Here's how the part is built. I have some questions about the finished solid (model axes, mm). A direction names the side the tool comes from. Round coordinates to 2 decimals unless told otherwise and drop trailing zeros. Order: outer loops, then holes, each group sorted by start corner. A loop starts at its lowest first (then second) coordinate and runs counter-clockwise, first axis right, second up.
Autodesk Inventor part; units mm, degrees
ref_plane "YZ Plane" through (0, 0, 0) normal (1, 0, 0) x (0, 1, 0)
ref_plane "XZ Plane" through (0, 0, 0) normal (0, 1, 0) x (-1, 0, 0)
ref_plane "XY Plane" through (0, 0, 0) normal (0, 0, 1) x (1, 0, 0)
sketch "Sketch1" plane through (0, 0, 0) normal (0, 0, 1) x (1, 0, 0)
  circle A0 centre (0, 0) radius 3.5
  line L0 (77.9423, 0) -> (38.9711, -67.5)
  line L1 (38.9711, -67.5) -> (-38.9711, -67.5)
  line L2 (-38.9711, -67.5) -> (-77.9423, 0)
  line L3 (-77.9423, 0) -> (-38.9711, 67.5)
  line L4 (-38.9711, 67.5) -> (38.9711, 67.5)
  line L5 (38.9711, 67.5) -> (77.9423, 0)
  circle A1 centre (22.5, 0) radius 2.25
  circle A2 centre (54, 0) radius 2
  circle A3 centre (15.9099, 15.9099) radius 2.25
  circle A4 centre (0, 22.5) radius 2.25
  circle A5 centre (-15.9099, 15.9099) radius 2.25
  circle A6 centre (-22.5, 0) radius 2.25
  circle A7 centre (-15.9099, -15.9099) radius 2.25
  circle A8 centre (0, -22.5) radius 2.25
  circle A9 centre (15.9099, -15.9099) radius 2.25
  circle A10 centre (46.7654, 27) radius 2
  circle A11 centre (27, 46.7654) radius 2
  circle A12 centre (0, 54) radius 2
  circle A13 centre (-27, 46.7654) radius 2
  circle A14 centre (-46.7654, 27) radius 2
  circle A15 centre (-54, 0) radius 2
  circle A16 centre (-46.7654, -27) radius 2
  circle A17 centre (-27, -46.7654) radius 2
  circle A18 centre (0, -54) radius 2
  circle A19 centre (27, -46.7654) radius 2
  circle A20 centre (46.7654, -27) radius 2
  dimension "d0" = 7
  dimension "d1" = 135
  dimension "d2" = 22.5
  dimension "d3" = 4.5
  dimension "d4" = 4
  dimension "d5" = 54
  dimension "d8" = 360
  dimension "d12" = 360
extrude "Extrusion1" add sketch "Sketch1" along normal blind 30
sketch "Sketch2" plane through (0, 0, 30) normal (0, 0, 1) x (1, 0, 0)
  circle A0 centre (0, 0) radius 3.5
  circle A1 centre (0, 0) radius 49
  dimension "d16" = 98
extrude "Extrusion2" cut sketch "Sketch2" against normal blind 15
sketch "Sketch3" plane through (0, 0, 15) normal (0, 0, 1) x (1, 0, 0)
  circle A0 centre (0, 0) radius 33
  dimension "d19" = 66
extrude "Extrusion3" cut sketch "Sketch3" against normal blind 3
sketch "Sketch4" plane through (0, 0, 12) normal (0, 0, 1) x (1, 0, 0)
  circle A0 centre (0, 0) radius 16.5
  circle A1 centre (0, 0) radius 3.5
  dimension "d22" = 33
extrude "Extrusion4" add sketch "Sketch4" along normal blind 33
sketch "Sketch5" plane through (0, 0, 45) normal (0, 0, 1) x (1, 0, 0)
  circle A0 centre (8, 0) radius 2.5
  circle A1 centre (2.4721, 7.6085) radius 2.5
  circle A2 centre (-6.4721, 4.7023) radius 2.5
  circle A3 centre (-6.4721, -4.7023) radius 2.5
  circle A4 centre (2.4721, -7.6085) radius 2.5
  point P0 (0, 0)
  dimension "d25" = 5
  dimension "d26" = 8
  dimension "d29" = 360
extrude "Extrusion5" cut sketch "Sketch5" against normal through all
sketch "Sketch6" plane through (0, 0, 0) normal (0, 0, -1) x (-1, 0, 0)
  circle A0 centre (0, 0) radius 17.5
  dimension "d33" = 35
extrude "Extrusion6" cut sketch "Sketch6" against normal blind 5
sketch "Sketch10" plane through (0, 0, 0) normal (0, 0, -1) x (-1, 0, 0)
  circle A0 centre (22.5, 0) radius 2.25
  circle A1 centre (0, 0) radius 3.5
  circle A2 centre (0, 0) radius 20.25
  circle A3 centre (0, 0) radius 24.75
  circle A4 centre (0, 0) radius 16
  circle A5 centre (0, 0) radius 29
  line L0 (29, 0) -> (16, 0)
  dimension "d38" = 13
extrude "Extrusion7" cut sketch "Sketch10" against normal blind 5 contours L0 A0 | A2 | A3 | A5 | A0 L0
sketch "Sketch11" plane through (0, 0, 12) normal (0, 0, 1) x (1, 0, 0)
  circle A0 centre (0, 0) radius 16.5
  circle A1 centre (15.9099, -15.9099) radius 2.25
  circle A2 centre (0, -22.5) radius 2.25
  circle A3 centre (-15.9099, -15.9099) radius 2.25
  circle A4 centre (-22.5, 0) radius 2.25
  circle A5 centre (-15.9099, 15.9099) radius 2.25
  circle A6 centre (0, 22.5) radius 2.25
  circle A7 centre (15.9099, 15.9099) radius 2.25
  circle A8 centre (22.5, 0) radius 2.25
  circle A9 centre (0, 0) radius 33
extrude "Extrusion8" add sketch "Sketch11" along normal up to surface (3 mm away) from surface at 0
sketch "Sketch12" plane through (0, 0, 30) normal (0, 0, 1) x (1, 0, 0)
  circle A0 centre (0, 0) radius 49
  circle A1 centre (46.7654, -27) radius 2
  circle A2 centre (27, -46.7654) radius 2
  circle A3 centre (0, -54) radius 2
  circle A4 centre (-27, -46.7654) radius 2
  circle A5 centre (-46.7654, -27) radius 2
  circle A6 centre (-54, 0) radius 2
  circle A7 centre (-46.7654, 27) radius 2
  circle A8 centre (-27, 46.7654) radius 2
  circle A9 centre (0, 54) radius 2
  circle A10 centre (27, 46.7654) radius 2
  circle A11 centre (46.7654, 27) radius 2
  circle A12 centre (54, 0) radius 2
  line L0 (38.9711, -67.5) -> (77.9423, 0)
  line L1 (77.9423, 0) -> (38.9711, 67.5)
  line L2 (38.9711, 67.5) -> (-38.9711, 67.5)
  line L3 (-38.9711, 67.5) -> (-77.9423, 0)
  line L4 (-77.9423, 0) -> (-38.9711, -67.5)
  line L5 (-38.9711, -67.5) -> (38.9711, -67.5)
extrude "Extrusion9" cut sketch "Sketch12" against normal blind 1
sketch "Sketch14" plane through (0, 0, 15) normal (0, 0, 1) x (1, 0, 0)
  circle A0 centre (0, 0) radius 3.5
  circle A1 centre (0, 0) radius 33
  circle A2 centre (15.9099, -15.9099) radius 2.25
  circle A3 centre (0, -22.5) radius 2.25
  circle A4 centre (-15.9099, -15.9099) radius 2.25
  circle A5 centre (-22.5, 0) radius 2.25
  circle A6 centre (-15.9099, 15.9099) radius 2.25
  circle A7 centre (0, 22.5) radius 2.25
  circle A8 centre (15.9099, 15.9099) radius 2.25
  circle A9 centre (22.5, 0) radius 2.25
  circle A10 centre (0, 0) radius 16.5
  circle A11 centre (0, 0) radius 49
  dimension "d45" = 66
extrude "Extrusion10" cut sketch "Sketch14" against normal blind 4 contours A11
sketch "Sketch15" plane through (0, 0, 29) normal (0, 0, 1) x (1, 0, 0)
  circle A0 centre (0, 0) radius 49 construction
  circle A1 centre (54, 0) radius 2 construction
  circle A2 centre (46.7654, 27) radius 2 construction
  circle A3 centre (27, 46.7654) radius 2 construction
  circle A4 centre (0, 54) radius 2 construction
  circle A5 centre (-27, 46.7654) radius 2 construction
  circle A6 centre (-46.7654, 27) radius 2 construction
  circle A7 centre (-54, 0) radius 2 construction
  circle A8 centre (-46.7654, -27) radius 2 construction
  circle A9 centre (-27, -46.7654) radius 2 construction
  circle A10 centre (0, -54) radius 2 construction
  circle A11 centre (27, -46.7654) radius 2 construction
  circle A12 centre (46.7654, -27) radius 2 construction
  line L0 (77.9423, 0) -> (38.9711, -67.5)
  line L1 (38.9711, 67.5) -> (77.9423, 0)
  line L2 (-38.9711, 67.5) -> (38.9711, 67.5)
  line L3 (-77.9423, 0) -> (-38.9711, 67.5)
  line L4 (-38.9711, -67.5) -> (-77.9423, 0)
  line L5 (38.9711, -67.5) -> (-38.9711, -67.5)
  line L6 (36.0844, 62.5) -> (72.1688, 0)
  line L7 (72.1688, 0) -> (36.0844, -62.5)
  line L8 (36.0844, -62.5) -> (-36.0844, -62.5)
  line L9 (-36.0844, -62.5) -> (-72.1688, 0)
  line L10 (-72.1688, 0) -> (-36.0844, 62.5)
  line L11 (-36.0844, 62.5) -> (36.0844, 62.5)
  dimension "d48" = 5
extrude "Extrusion11" add sketch "Sketch15" along normal blind 0.8
sketch "Sketch16" plane through (0, 0, 0) normal (0, 0, -1) x (-1, 0, 0)
  circle A0 centre (0, 0) radius 29
  circle A1 centre (-46.7654, -27) radius 2
  circle A2 centre (-27, -46.7654) radius 2
  circle A3 centre (0, -54) radius 2
  circle A4 centre (27, -46.7654) radius 2
  circle A5 centre (46.7654, -27) radius 2
  circle A6 centre (54, 0) radius 2
  circle A7 centre (46.7654, 27) radius 2
  circle A8 centre (27, 46.7654) radius 2
  circle A9 centre (0, 54) radius 2
  circle A10 centre (-27, 46.7654) radius 2
  circle A11 centre (-46.7654, 27) radius 2
  circle A12 centre (-54, 0) radius 2
  line L0 (-77.9423, 0) -> (-38.9711, -67.5)
  line L1 (-38.9711, -67.5) -> (38.9711, -67.5)
  line L2 (38.9711, -67.5) -> (77.9423, 0)
  line L3 (77.9423, 0) -> (38.9711, 67.5)
  line L4 (38.9711, 67.5) -> (-38.9711, 67.5)
  line L5 (-38.9711, 67.5) -> (-77.9423, 0)
  line L6 (68.1273, 0) -> (34.0637, -59)
  line L7 (34.0637, -59) -> (-34.0637, -59)
  line L8 (-34.0637, -59) -> (-68.1273, 0)
  line L9 (-68.1273, 0) -> (-34.0637, 59)
  line L10 (-34.0637, 59) -> (34.0637, 59)
  line L11 (34.0637, 59) -> (68.1273, 0)
  dimension "d51" = 118
extrude "Extrusion12" cut sketch "Sketch16" along normal through all both and the other way through all contours L5 L4 L3 L2 L1 L0
sketch "Sketch17" plane through (0, 0, 0) normal (0, 0, -1) x (-1, 0, 0)
  circle A0 centre (0, -54) radius 2
  circle A1 centre (0, -54) radius 2
  circle A2 centre (27, -46.7654) radius 2
  circle A3 centre (46.7654, -27) radius 2
  circle A4 centre (54, 0) radius 2
  circle A5 centre (46.7654, 27) radius 2
  circle A6 centre (27, 46.7654) radius 2
  circle A7 centre (0, 54) radius 2
  circle A8 centre (-27, 46.7654) radius 2
  circle A9 centre (-46.7654, 27) radius 2
  circle A10 centre (-54, 0) radius 2
  circle A11 centre (-46.7654, -27) radius 2
  circle A12 centre (-27, -46.7654) radius 2
  point P0 (0, 0)
  dimension "d56" = 360
extrude "Extrusion13" add sketch "Sketch17" along normal up to surface (29 mm away) from surface at -29
sketch "Sketch18" plane through (0, 0, 0) normal (0, 0, -1) x (-1, 0, 0)
  line L0 (-46.188, 0) -> (-23.094, 40)
  line L1 (-23.094, 40) -> (23.094, 40)
  line L2 (23.094, 40) -> (46.188, 0)
  line L3 (46.188, 0) -> (23.094, -40)
  line L4 (23.094, -40) -> (-23.094, -40)
  line L5 (-23.094, -40) -> (-46.188, 0)
  line L6 (-19.0526, -33) -> (19.0526, -33)
  line L7 (19.0526, -33) -> (38.1051, 0)
  line L8 (38.1051, 0) -> (19.0526, 33)
  line L9 (19.0526, 33) -> (-19.0526, 33)
  line L10 (-19.0526, 33) -> (-38.1051, 0)
  line L11 (-38.1051, 0) -> (-19.0526, -33)
  line L12 (-34.0637, -59) -> (34.0637, -59)
  line L13 (34.0637, -59) -> (68.1273, 0)
  line L14 (68.1273, 0) -> (34.0637, 59)
  line L15 (34.0637, 59) -> (-34.0637, 59)
  line L16 (-34.0637, 59) -> (-68.1273, 0)
  line L17 (-68.1273, 0) -> (-34.0637, -59)
  circle A0 centre (0, 0) radius 29
  dimension "d60" = 80
  dimension "d61" = 7
extrude "Extrusion14" add sketch "Sketch18" along normal blind 13 contours L0 L1 L2 L3 L4 L5 | L17 L16 L15 L14 L13 L12
sketch "Sketch19" plane through (68.1273, 0, 29) normal (0.866, 0.5, 0) x (0, 0, -1)
  line L0 (29, 15.0111) -> (29, 53.1162)
  line L1 (29, 15.0111) -> (42, 15.0111)
  line L2 (42, 53.1162) -> (42, 15.0111)
  line L3 (29, 53.1162) -> (42, 53.1162)
  line L4 (38, 26.9926) -> (33, 41.1347) construction
  circle A0 centre (38, 26.9926) radius 2.5
  circle A1 centre (33, 41.1347) radius 2.5
  point P0 (29, 34.0637)
  point P1 (35.5, 15.0111)
  point P2 (35.5, 34.0637)
  point P3 (29, 34.0637)
  dimension "d64" = 15
  dimension "d65" = 5
  dimension "d66" = 5
  dimension "d72" = 5
extrude "Extrusion15" cut sketch "Sketch19" against normal blind 30 contours A0 | A1
pattern_circular "Circular Pattern1" count 6 over 360 about axis through (0, 0, 0) along (0, 0, 1) of "Extrusion15"
sketch "Sketch21" plane through (0, 0, 5) normal (0, 0, -1) x (-1, 0, 0)
  circle A0 centre (0, 17.5) radius 2
  circle A1 centre (-15.1554, -8.75) radius 2
  circle A2 centre (15.1554, -8.75) radius 2
  point P0 (0, 0)
  dimension "d74" = 4
  dimension "d75" = 17.5
  dimension "d78" = 360
extrude "Extrusion16" cut sketch "Sketch21" against normal through all
sketch "Sketch22" plane through (0, 0, 5) normal (0, 0, -1) x (-1, 0, 0)
  circle A0 centre (-15.1554, -8.75) radius 2
  circle A1 centre (0, 17.5) radius 2
  circle A2 centre (15.1554, -8.75) radius 2
  circle A3 centre (0, 0) radius 29
  circle A4 centre (-22.5, 0) radius 2.25
  circle A5 centre (-15.9099, 15.9099) radius 2.25
  circle A6 centre (0, 22.5) radius 2.25
  circle A7 centre (15.9099, 15.9099) radius 2.25
  circle A8 centre (22.5, 0) radius 2.25
  circle A9 centre (15.9099, -15.9099) radius 2.25
  circle A10 centre (0, -22.5) radius 2.25
  circle A11 centre (-15.9099, -15.9099) radius 2.25
  circle A12 centre (0, 0) radius 3.5
extrude "Extrusion17" cut sketch "Sketch22" against normal blind 5
sketch "Sketch23" plane through (0, 0, 10) normal (0, 0, -1) x (-1, 0, 0)
  circle A0 centre (0, 0) radius 3.5
  circle A1 centre (0, 0) radius 14.5
  dimension "d84" = 29
extrude "Extrusion18" [suppressed]
sketch "Sketch24" plane through (0, 0, 29) normal (0, 0, 1) x (1, 0, 0)
  line L0 (-34.0637, -59) -> (34.0637, -59)
  line L1 (34.0637, -59) -> (68.1273, 0)
  line L2 (68.1273, 0) -> (34.0637, 59)
  line L3 (34.0637, 59) -> (-34.0637, 59)
  line L4 (-34.0637, 59) -> (-68.1273, 0)
  line L5 (-68.1273, 0) -> (-34.0637, -59)
  circle A0 centre (0, 0) radius 49
extrude "Extrusion19" add sketch "Sketch24" along normal blind 1
sketch "Sketch25" plane through (0, 0, 10) normal (0, 0, -1) x (-1, 0, 0)
  circle A0 centre (-15.1554, -8.75) radius 2
  circle A1 centre (0, 17.5) radius 2
  circle A2 centre (15.1554, -8.75) radius 2
  point P0 (0, 0)
extrude "Extrusion20" add sketch "Sketch25" against normal up to surface (5 mm away) from surface at 0
sketch "Sketch26" plane through (0, 0, -13) normal (0, 0, -1) x (-1, 0, 0)
  circle A0 centre (-62, 0) radius 2.25
  circle A1 centre (-31, -53.6936) radius 2.25
  circle A2 centre (31, -53.6936) radius 2.25
  circle A3 centre (62, 0) radius 2.25
  circle A4 centre (31, 53.6936) radius 2.25
  circle A5 centre (-31, 53.6936) radius 2.25
  point P0 (0, 0)
  dimension "d91" = 4.5
  dimension "d92" = 62
  dimension "d95" = 360
extrude "Extrusion21" cut sketch "Sketch26" against normal through all
properties part number "AC05" material "ABS Plastic"
1. If we section it at D-D, the plane z = 33.5: Write out the boundary of the cut face in (x, y).
Evaluation:
outline: (-15.06, -6.75) arc R2 cw to (-13.38, -9.66) arc R16.5 ccw to (13.38, -9.66) arc R2 cw to (15.06, -6.75) arc R16.5 ccw to (1.68, 16.41) arc R2 cw to (-1.68, 16.41) arc R16.5 ccw to start; hole circle Ø5 at (-6.47, -4.7); hole circle Ø5 at (-6.47, 4.7); hole circle Ø7 at (0, 0); hole circle Ø5 at (2.47, -7.61); hole circle Ø5 at (2.47, 7.61); hole circle Ø5 at (8, 0)
2. On a 3-axis mill with a long thin cutter (end or side, diameter ignored), from which of +Z, -Z, +X, -X, +Y, -Y can I reach the whole of each face in a straight line? I mean faces 3 (the cylindrical face through (-9.51, -46.18, -8.46)), 4 (the cylindrical face through (-13.437, -7.726, 29.79)), 5 (the flat face through (0, -6, 10)). Say none if no direction works.
Evaluation:
face 3: -Y
face 4: +Z
face 5: -Z
3. If we section it at B-B, the plane x = -22: Write out the boundary of the cut face in (y, z).
Evaluation:
outline: (-59, -13) - (-27.89, -13) - (-27.89, 0) - (-18.89, 0) - (-18.89, 10) - (-2.19, 10) - (-2.19, 15) - (-24.6, 15) - (-24.6, 11) - (-43.78, 11) - (-43.78, 30) - (-59, 30) - close; (2.19, 10) - (18.89, 10) - (18.89, 0) - (27.89, 0) - (27.89, -13) - (59, -13) - (59, 30) - (43.78, 30) - (43.78, 11) - (24.6, 11) - (24.6, 15) - (2.19, 15) - close
4. If we section it at C-C, the plane y = -42: Write out the boundary of the cut face in (x, z), and give its area (3 significant figures).
Evaluation:
outline: (-43.88, -13) - (43.88, -13) - (43.88, 30) - (25.24, 30) - (25.24, 11) - (-25.24, 11) - (-25.24, 30) - (-43.88, 30) - close; hole circle Ø5 at (-7.07, -9); hole circle Ø5 at (7.07, -4)
area: 2,780 mm2
5. I need wall thicknesses on probe 1 along Y at (x, z) = (31, 7); probe 2 along X at (y, z) = (6, 36); probe 3 along Y at (x, z) = (17, -0.5). Which ranges of each line are inside material? Lowest first, please.
Evaluation:
probe 1: y = -59 to -55.94, -51.44 to 51.44, 55.94 to 59
probe 2: x = -15.37 to -8.61, -4.34 to 0.56, 4.39 to 15.37
probe 3: y = -59 to -33, 33 to 59
6. If we section it at A-A, the plane z = 20: State how many separate pieces and enclosed holes the cut face has, and give its area (3 significant figures).
Evaluation:
separate pieces: 2
enclosed holes: 13
area: 5,130 mm2
7. If we mould it in two halves opening along X, with no side actions, what happens to faces 1 (the flat face through (0, 4, 45)), 2 (the cylindrical face through (13.41, -7.77, 29.79))? For each: released by +X, released by -X, zero draft, split by the parting line, or undercut.
Evaluation:
face 1: zero draft
face 2: undercut
8. I'm going to push flat-ended pins straight in: P1, Ø3, axis at y = -26, z = 0, coming from the -X side; P2, Ø6, axis at x = 17, y = -19, coming from the +Z side; P3, Ø1, axis at y = -9, z = 34.5, coming from the +X side; P4, Ø4.5, axis at x = 8, y = 0, coming from the +Z side. Where does each tip first touch, or does it pass through?
Evaluation:
P1: stops at x = -53.98
P2: stops at z = 15
P3: stops at x = 13.3
P4: passes through
